```python
from build123d import *

# Parameters (mm, degrees)
F1_DEPTH = 66.04
F2_W     = 58.42
F2_H     = 71.12
F3_DEPTH = 3.81
F4_W     = 58.42
F4_H     = 12.7
F5_DEPTH = 101.6
F6_W     = 58.42
F6_H     = 68.58
F7_DEPTH = 25.4


with BuildPart() as f1:
    # F0 (on Right) → F1 (new body)
    with BuildSketch(Plane.YZ):
        Polygon((-79.753995, 36.364574), (-77.213995, 16.044574), (-1.013995, 16.044574), (-1.013995, 36.364574), align=None)
        Polygon((-75.438095, 32.554574), (-4.823995, 32.554574), (-4.823995, 19.651505), (-73.825211, 19.651505), align=None, mode=Mode.SUBTRACT)
    extrude(amount=F1_DEPTH)

    # F2 (on face) → F3 (cut)
    with BuildSketch(Plane.XY.offset(36.364574)):
        with Locations((33.02, -40.383995)):
            Rectangle(F2_W, F2_H)
    extrude(amount=-F3_DEPTH, mode=Mode.SUBTRACT)

    # F4 (on face) → F5 (cut)
    with BuildSketch(Plane(origin=(0, -1.013995, 0), x_dir=(-1, 0, 0), z_dir=(0, 1, 0))):
        with Locations((-33.02, 26.204574)):
            Rectangle(F4_W, F4_H)
    extrude(amount=-F5_DEPTH, mode=Mode.SUBTRACT)

    # F6 (on face) → F7 (cut)
    with BuildSketch(Plane(origin=(0, 0, 16.044574), x_dir=(1, 0, 0), z_dir=(0, 0, -1))):
        with Locations((33.02, 39.113995)):
            Rectangle(F6_W, F6_H)
    extrude(amount=-F7_DEPTH, mode=Mode.SUBTRACT)


solid = f1.part
```
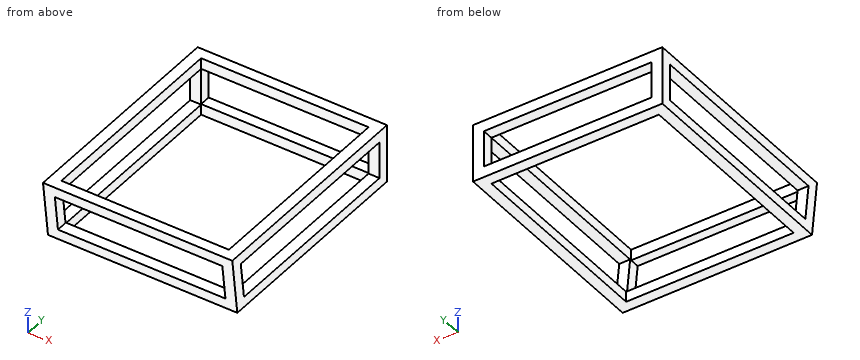
Check sheet for the modelled part. Datum: model origin and axes. Units: mm. Round coordinates to 2 decimals unless told otherwise and drop trailing zeros. Write each loop counter-clockwise with the first axis right and the second up, starting at its lowest first coordinate (ties: lowest second). Pieces come first, ordered by that corner, then holes. Notation, with made-up numbers: (43.5, 42) -> (62.5, 42) arc R32 ccw to (62.5, 80) -> close; hole circle Ø11 at (39.25, 63). An arc over 180 degrees is marked (long way). One line per question, with ' | ' between items. Start each with the question number.
1. Sectioned sample at C-C, the plane z = 34.5. Record the cut outline in (x, y).
2. Sectioned sample at D-D, the plane z = 21.5. Record the cut outline in (x, y), then the cut area to 3 significant figures.
3. Scan lines: line 1 along X through (y, z) = (-21, 19); line 2 along Y through (x, z) = (43.5, 33.5); line 3 along Y through (x, z) = (3, 23.5). Record each from-to range of solid material in increasing order. Write a range as from..to.
4. Depth check by flat-ended pin: pin 1 (5 mm diameter, centred on x = 31, z = 21.5, fed in from -Y); pin 2 (8 mm diameter, centred on x = 23, z = 25, fed in from -Y); pin 3 (1.1 mm diameter, centred on x = 31.5, z = 35, fed in from -Y); pin 4 (4 mm diameter, centred on x = 7.5, z = 32, fed in from -Y). Enter the tip coordinate at first touch or a pass-through.
5. Sectioned sample at B-B, the plane y = -12.5. Record the cut outline in (x, z).
6. Sectioned sample at A-A, the plane x = 20. Record the cut outline in (y, z), then the cut area to 3 significant figures.
Taken from the geometry:
1) outline: (0, -79.52) -> (66.04, -79.52) -> (66.04, -1.01) -> (0, -1.01) -> close; hole (3.81, -75.94) -> (62.23, -75.94) -> (62.23, -4.82) -> (3.81, -4.82) -> close
2) outline: (0, -77.9) -> (3.81, -77.9) -> (3.81, -74.06) -> (0, -74.06) -> close; (0, -4.82) -> (3.81, -4.82) -> (3.81, -1.01) -> (0, -1.01) -> close; (62.23, -77.9) -> (66.04, -77.9) -> (66.04, -74.06) -> (62.23, -74.06) -> close; (62.23, -4.82) -> (66.04, -4.82) -> (66.04, -1.01) -> (62.23, -1.01) -> close | area: 58.3 mm^2
3) line 1: x = 0..3.81, 62.23..66.04 | line 2: y = -79.4..-75.94, -4.82..-1.01 | line 3: y = -78.15..-74.31, -4.82..-1.01
4) pin 1: stops at y = -77.69 | pin 2: passes through | pin 3: stops at y = -79.65 | pin 4: stops at y = -79.46
5) outline: (0, 16.04) -> (3.81, 16.04) -> (3.81, 19.65) -> (0, 19.65) -> close; (0, 32.55) -> (3.81, 32.55) -> (3.81, 36.36) -> (0, 36.36) -> close; (62.23, 16.04) -> (66.04, 16.04) -> (66.04, 19.65) -> (62.23, 19.65) -> close; (62.23, 32.55) -> (66.04, 32.55) -> (66.04, 36.36) -> (62.23, 36.36) -> close
6) outline: (-79.75, 36.36) -> (-79.28, 32.55) -> (-75.94, 32.55) -> (-75.94, 36.36) -> close; (-77.69, 19.85) -> (-77.21, 16.04) -> (-73.4, 16.04) -> (-73.4, 19.65) -> (-73.83, 19.65) -> (-73.85, 19.85) -> close; (-4.82, 16.04) -> (-1.01, 16.04) -> (-1.01, 19.85) -> (-4.82, 19.85) -> close; (-4.82, 32.55) -> (-1.01, 32.55) -> (-1.01, 36.36) -> (-4.82, 36.36) -> close | area: 58.0 mm^2
